```python
from build123d import *

# Parameters (mm, degrees)
SPHERE_ANGLE      = 180
CYLINDER184_R     = 2.5
CYLINDER184_DEPTH = 6.2


with BuildPart() as obj1_sphere:
    # Sphere → Sphere (revolve)
    with BuildSketch(Plane(origin=(0, 0, 6.2), x_dir=(1, 0, 0), z_dir=(0, 0, -1))):
        with BuildLine():
            ThreePointArc((0, -2.5), (2.5, 0), (0, 2.5))
            Line((0, 2.5), (0, -2.5))
        make_face()
    revolve(axis=Axis((0, 0, 6.2), (0, -1, 0)), revolution_arc=SPHERE_ANGLE)


with BuildPart() as obj1:
    # Cylinder184 → Cylinder184 (new body)
    with BuildSketch(Plane.XY):
        Circle(CYLINDER184_R)
    extrude(amount=CYLINDER184_DEPTH)

    # Fusion005: union obj1_sphere
    add(obj1_sphere.part)


solid = obj1.part
```
Here's how the part is built. I have some questions about the finished solid (model axes, mm). Coordinates: 2 decimals unless noted, no trailing zeros. Write each loop counter-clockwise with the first axis right and the second up, starting at its lowest first coordinate (ties: lowest second). Pieces come first, ordered by that corner, then holes. Notation, with made-up numbers: (64, 64.25) -> (117, 64.25) arc R36 ccw to (117, 103.25) -> close; hole circle Ø10 at (20.5, 72.25). An arc over 180 degrees is marked (long way). Use a Markdown table: item, result. Add a question column.
(1) I'm going to push a flat-ended pin straight in: P1, Ø2, axis at x = 1.5, y = 1, coming from the +Z side. Where does the tip first touch, or does it pass through?
(2) If we section it at C-C, the plane z = 1.5: Write out the boundary of the cut face in (x, y).
(3) Please list where these lines run through material, in increasing order: line 1 (Y direction, x = 0.6, z = 6.25); line 2 (X direction, y = 1.8, z = 6); line 3 (X direction, y = 1.45, z = 4.5).
(4) If we section it at A-A, the plane y = -1.5: Write out the boundary of the cut face in (x, z).
(5) If we section it at D-D, the plane z = 6.5: Write out the boundary of the cut face in (x, y).
Outcome:
| question | item | result |
|---|---|---|
| 1 | P1 | stops at z = 8.57 |
| 2 | outline | circle Ø5 at (0, 0) |
| 3 | line 1 | y = -2.43 to 2.43 |
| 3 | line 2 | x = -1.73 to 1.73 |
| 3 | line 3 | x = -2.04 to 2.04 |
| 4 | outline | (-2, 0) -> (2, 0) -> (2, 6.2) arc R2 ccw to (-2, 6.2) -> close |
| 5 | outline | circle Ø4.96 at (0, 0) |
